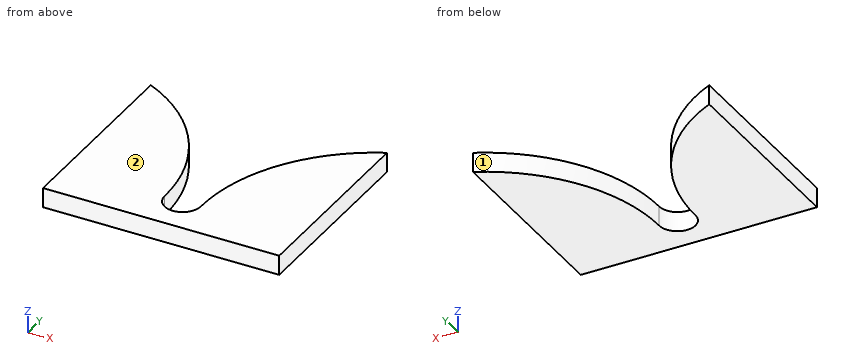
from build123d import *

# Parameters (mm, degrees)
BOSS_EXTRUDE2_DEPTH = 3.175


with BuildPart() as part:
    # Sketch1 → Boss-Extrude2 (new, symmetric)
    with BuildSketch(Plane.XY):
        with BuildLine():
            Line((76.2, 0), (76.2, 6.35))
            Line((76.2, 6.35), (76.2, 63.5))
            ThreePointArc((76.2, 63.5), (52.687880643, 42.788280792), (43.942, 12.7))
            ThreePointArc((43.942, 12.7), (38.1, 6.858), (32.258, 12.7))
            ThreePointArc((32.258, 12.7), (23.512119357, 42.788280792), (0, 63.5))
            Line((0, 63.5), (0, 6.35))
            Line((0, 6.35), (0, 0))
            Line((0, 0), (76.2, 0))
        make_face()
    extrude(amount=BOSS_EXTRUDE2_DEPTH, both=True)


solid = part.part
For this review, take the finished solid that the model builds, in its own axes (mm). Face numbers are marked on the shaded views. Round coordinates to 2 decimals unless told otherwise and drop trailing zeros. Write each loop counter-clockwise with the first axis right and the second up, starting at its lowest first coordinate (ties: lowest second). Pieces come first, ordered by that corner, then holes. Notation, with made-up numbers: M -19.5,44 L -13.5,44 A27 ccw -13.5,63 Z; hole C 20,-11.75 d6. An arc over 180 degrees is marked long. Write item = value, one per line. Start each with the question number.
(1) We need section B-B (x = 38.1). Give the boundary of the cut face in (y, z) (3 decimals).
(2) The part is to be moulded in two halves that separate along X. For the marked faces 1 and 2, say which applies: +X half, -X half, draft (parallel to the pull), parting line (faces both ways), or undercut.
(3) We need section C-C (z = 1.25). Give the boundary of the cut face in (x, y).
(4) We need section A-A (y = 52.5). Give the boundary of the cut face in (x, z) (3 decimals), then the cut area to 3 significant figures.
(5) Clearance check with a flat-ended pin moving along its axis: pin 1 Ø10 at (x, y) = (39, 31) entering from +Z. State where the tip first meets the part, or that it passes through.
(6) For line 1 along X through (y, z) = (23, -0.5); line 2 along X through (y, z) = (55.5, -1); line 3 along Y through (x, z) = (53.5, 0.5), list the stretches that pass through material, from the lowest coordinate up.
(7) We need section D-D (x = 6). Give the boundary of the cut face in (y, z) (3 decimals).
Results found:
q1.outline = M 0,-3.175 L 6.858,-3.175 L 6.858,3.175 L 0,3.175 Z
q2.face_1 = undercut
q2.face_2 = draft
q3.outline = M 0,0 L 76.2,0 L 76.2,63.5 A56.13 ccw 43.94,12.7 A5.84 cw 32.26,12.7 A56.13 ccw 0,63.5 Z
q4.outline = M 0,-3.175 L 15.707,-3.175 L 15.707,3.175 L 0,3.175 Z; M 60.493,-3.175 L 76.2,-3.175 L 76.2,3.175 L 60.493,3.175 Z
q4.area = 199 mm²
q5.pin_1 = through
q6.line_1 = 0 to 31.3, 44.9 to 76.2
q6.line_2 = 0 to 12.44, 63.76 to 76.2
q6.line_3 = 0 to 44.03
q7.outline = M 0,-3.175 L 60.22,-3.175 L 60.22,3.175 L 0,3.175 Z
